The figure shows three views and two pictorial views of one solid part (mm, origin at its lowest corner). Answer the questions. Round coordinates to 2 decimals unless told otherwise and drop trailing zeros. Order: outer loops, then holes, each group sorted by start corner. A loop starts at its lowest first (then second) coordinate and runs counter-clockwise, first axis right, second up. Notation, with made-up numbers: (44.25, 63.5) - (71.25, 63.5) arc R9 ccw to (71.25, 71.5) - close; hole circle Ø6 at (-1.75, 75.25). An arc over 180 degrees is marked (long way). Write item = value, one per line.
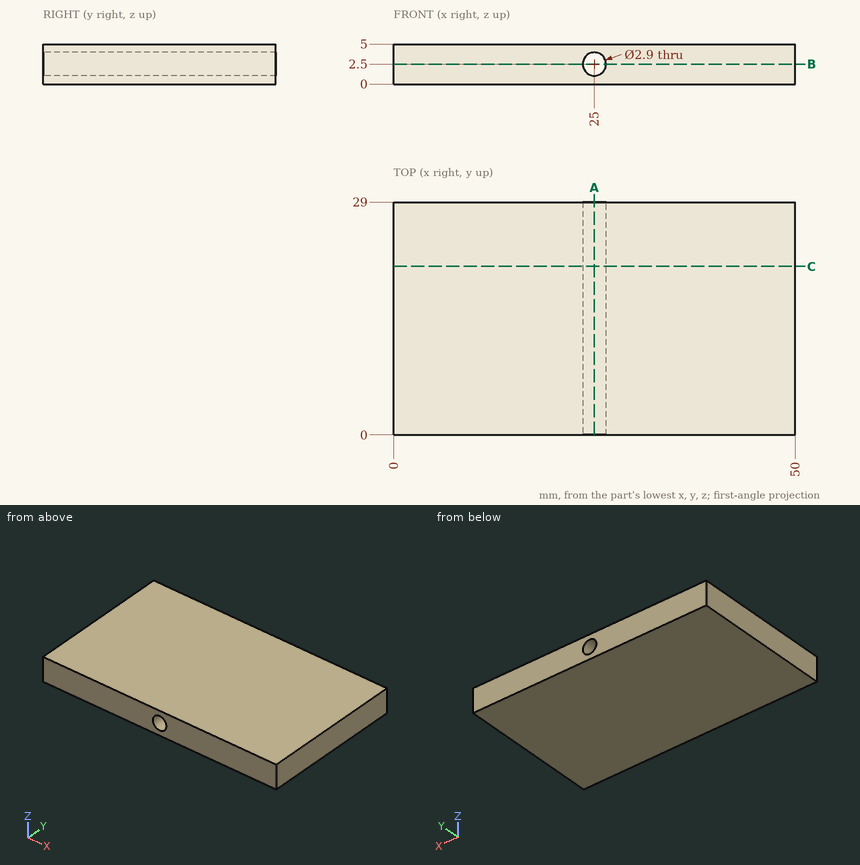
Q1. Section C-C on y = 21 is taken. Determine the outline of the cut face in (x, z).
Model answer:
outline = (0, 0) - (50, 0) - (50, 5) - (0, 5) - close; hole circle Ø2.9 at (25, 2.5)
Q2. Section B-B on z = 2.5 is taken. Determine the outline of the cut face in (x, y).
Model answer:
outline = (0, 0) - (23.55, 0) - (23.55, 29) - (0, 29) - close; (26.45, 0) - (50, 0) - (50, 29) - (26.45, 29) - close
Q3. Section A-A on x = 25 is taken. Determine the outline of the cut face in (y, z).
Model answer:
outline = (0, 0) - (29, 0) - (29, 1.05) - (0, 1.05) - close; (0, 3.95) - (29, 3.95) - (29, 5) - (0, 5) - close
Q4. A flat-ended cylindrical pin translates along its axis: P1, Ø1, axis at y = 10, z = 1, coming from the -X side. Find the tip coordinate at first contact, or state that the pin passes through.
Model answer:
P1 = 0
Q5. Find the intervals of material crossed by line 1 (Z direction, x = 25, y = 12.75); line 2 (X direction, y = 20.75, z = 1.4); line 3 (X direction, y = 21.25, z = 2.7), in increasing order. Write a range as from..to.
Model answer:
line_1 = 0..1.05, 3.95..5
line_2 = 0..24.06, 25.94..50
line_3 = 0..23.56, 26.44..50
